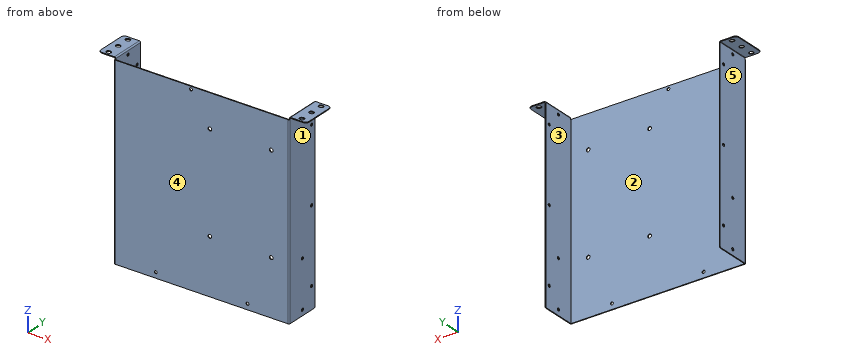
```python
from build123d import *

# Parameters (mm, degrees)
SKETCH1_W                    = 214
SKETCH1_H                    = 230.5
BASE_FLANGE1_DEPTH           = 1
EDGE_FLANGE3_STRIP_W         = 5
EDGE_FLANGE3_STRIP_H         = 1
EDGE_FLANGE3_STRIP_CUT_DEPTH = 230.5
EDGE_FLANGE3_DEPTH           = 230.5
EDGE_FLANGE4_STRIP_W         = 5
EDGE_FLANGE4_STRIP_H         = 1
EDGE_FLANGE4_STRIP_CUT_DEPTH = 230.5
EDGE_FLANGE4_DEPTH           = 230.5
EDGE_FLANGE5_STRIP_W         = 5
EDGE_FLANGE5_STRIP_H         = 1
EDGE_FLANGE5_STRIP_CUT_DEPTH = 41.5
EDGE_FLANGE5_DEPTH           = 41.5
EDGE_FLANGE6_STRIP_W         = 5
EDGE_FLANGE6_STRIP_H         = 1
EDGE_FLANGE6_STRIP_CUT_DEPTH = 41.5
EDGE_FLANGE6_DEPTH           = 41.5
FILLET1_R                    = 4
CUT_EXTRUDE1_REACH           = 178.807
SKETCH24_W                   = 214
SKETCH24_H                   = 2.5
SKETCH26_R                   = 2.5
CUT_EXTRUDE2_DEPTH           = 10
SKETCH27_R                   = 1.75
CUT_EXTRUDE3_DEPTH           = 265.201745831
SKETCH28_R                   = 2.25
CUT_EXTRUDE4_DEPTH           = 177.806568034
SKETCH29_R                   = 1.75
CUT_EXTRUDE5_DEPTH           = 177.566028726
SKETCH30_R                   = 1.75
CUT_EXTRUDE6_DEPTH           = 265.201745831
SKETCH31_R                   = 1.75
CUT_EXTRUDE7_DEPTH           = 265.201745831
CHAMFER1_SIZE                = 1
CUT_EXTRUDE8_DEPTH           = 266.637440885
SKETCH33_R                   = 1.75
CUT_EXTRUDE9_DEPTH           = 177.806568034
SKETCH34_R                   = 1.75
CUT_EXTRUDE10_DEPTH          = 265.201745831


# Sheet-metal steps are written as plain solids
with BuildPart() as part:
    # Sketch1 → Base-Flange1 (new body)
    with BuildSketch(Plane(origin=(0, 0, 0), x_dir=(1, 0, 0), z_dir=(0, 1, 0))):
        Rectangle(SKETCH1_W, SKETCH1_H)
    extrude(amount=-BASE_FLANGE1_DEPTH)

    # Edge-Flange3 strip (across the edge) → Edge-Flange3 strip cut (cut)
    with BuildSketch(Plane(origin=(-107, 0, -115.25), x_dir=(1, 0, 0), z_dir=(0, 0, 1))):
        with Locations((-1, -0.5)):
            Rectangle(EDGE_FLANGE3_STRIP_W, EDGE_FLANGE3_STRIP_H)
    extrude(amount=EDGE_FLANGE3_STRIP_CUT_DEPTH, mode=Mode.SUBTRACT)

    # Edge-Flange3 section (across the edge) → Edge-Flange3 (add)
    with BuildSketch(Plane(origin=(-107, 0, -115.25), x_dir=(1, 0, 0), z_dir=(0, 0, 1))):
        with BuildLine():
            Line((0, 0.5), (0, 42))
            Line((0, 42), (1, 42))
            Line((1, 42), (1, 0.5))
            ThreePointArc((1, 0.5), (1.146446609, 0.146446609), (1.5, 0))
            Line((1.5, 0), (1.5, -1))
            ThreePointArc((1.5, -1), (0.439339828, -0.560660172), (0, 0.5))
        make_face()
    extrude(amount=EDGE_FLANGE3_DEPTH)

    # Edge-Flange4 strip (across the edge) → Edge-Flange4 strip cut (cut)
    with BuildSketch(Plane(origin=(107, 0, 115.25), x_dir=(-1, 0, 0), z_dir=(0, 0, -1))):
        with Locations((-1, -0.5)):
            Rectangle(EDGE_FLANGE4_STRIP_W, EDGE_FLANGE4_STRIP_H)
    extrude(amount=EDGE_FLANGE4_STRIP_CUT_DEPTH, mode=Mode.SUBTRACT)

    # Edge-Flange4 section (across the edge) → Edge-Flange4 (add)
    with BuildSketch(Plane(origin=(107, 0, 115.25), x_dir=(-1, 0, 0), z_dir=(0, 0, -1))):
        with BuildLine():
            Line((0, 0.5), (0, 42))
            Line((0, 42), (1, 42))
            Line((1, 42), (1, 0.5))
            ThreePointArc((1, 0.5), (1.146446609, 0.146446609), (1.5, 0))
            Line((1.5, 0), (1.5, -1))
            ThreePointArc((1.5, -1), (0.439339828, -0.560660172), (0, 0.5))
        make_face()
    extrude(amount=EDGE_FLANGE4_DEPTH)

    # Edge-Flange5 strip (across the edge) → Edge-Flange5 strip cut (cut)
    with BuildSketch(Plane(origin=(107, 42, 115.25), x_dir=(0, 0, -1), z_dir=(0, -1, 0))):
        with Locations((-1, -0.5)):
            Rectangle(EDGE_FLANGE5_STRIP_W, EDGE_FLANGE5_STRIP_H)
    extrude(amount=EDGE_FLANGE5_STRIP_CUT_DEPTH, mode=Mode.SUBTRACT)

    # Edge-Flange5 section (across the edge) → Edge-Flange5 (add)
    with BuildSketch(Plane(origin=(107, 42, 115.25), x_dir=(0, 0, -1), z_dir=(0, -1, 0))):
        with BuildLine():
            Line((0, 0.5), (0, 20))
            Line((0, 20), (1, 20))
            Line((1, 20), (1, 0.5))
            ThreePointArc((1, 0.5), (1.146446609, 0.146446609), (1.5, 0))
            Line((1.5, 0), (1.5, -1))
            ThreePointArc((1.5, -1), (0.439339828, -0.560660172), (0, 0.5))
        make_face()
    extrude(amount=EDGE_FLANGE5_DEPTH)

    # Edge-Flange6 strip (across the edge) → Edge-Flange6 strip cut (cut)
    with BuildSketch(Plane(origin=(-107, 0.5, 115.25), x_dir=(0, 0, -1), z_dir=(0, 1, 0))):
        with Locations((-1, -0.5)):
            Rectangle(EDGE_FLANGE6_STRIP_W, EDGE_FLANGE6_STRIP_H)
    extrude(amount=EDGE_FLANGE6_STRIP_CUT_DEPTH, mode=Mode.SUBTRACT)

    # Edge-Flange6 section (across the edge) → Edge-Flange6 (add)
    with BuildSketch(Plane(origin=(-107, 0.5, 115.25), x_dir=(0, 0, -1), z_dir=(0, 1, 0))):
        with BuildLine():
            Line((0, 0.5), (0, 20))
            Line((0, 20), (1, 20))
            Line((1, 20), (1, 0.5))
            ThreePointArc((1, 0.5), (1.146446609, 0.146446609), (1.5, 0))
            Line((1.5, 0), (1.5, -1))
            ThreePointArc((1.5, -1), (0.439339828, -0.560660172), (0, 0.5))
        make_face()
    extrude(amount=EDGE_FLANGE6_DEPTH)

    # Fillet1
    fillet1_edges = [part.edges().sort_by_distance(p)[0] for p in [
        (127, 42, 114.75),
        (127, 0.5, 114.75),
        (-127, 0.5, 114.75),
        (-127, 42, 114.75),
    ]]
    fillet(fillet1_edges, radius=FILLET1_R)

    # Cut-Extrude1: up to this face of the body (flat: up to its plane)
    cut_extrude1_end = Plane(part.part.faces().sort_by_distance((114.980552593, 0.5, 114.747536063))[0])
    # Sketch24 → Cut-Extrude1 (cut, up to the picked face)
    with BuildSketch(Plane.XZ.offset(1), mode=Mode.PRIVATE) as cut_extrude1_sk1:
        with Locations((0, 114)):
            Rectangle(SKETCH24_W, SKETCH24_H)
    cut_extrude1_tool1 = split(extrude(cut_extrude1_sk1.sketch, amount=-CUT_EXTRUDE1_REACH, mode=Mode.PRIVATE), bisect_by=cut_extrude1_end, keep=Keep.BOTH, mode=Mode.PRIVATE)
    add(cut_extrude1_tool1.solids().sort_by(Axis((0, -1, 114), (0, 1, 0)))[0], mode=Mode.SUBTRACT)

    # Sketch26 → Cut-Extrude2 (cut)
    with BuildSketch(Plane.XY.offset(115.25)):
        with Locations((-118, 37)):
            Circle(SKETCH26_R)
        with Locations((-118, 5.24)):
            Circle(SKETCH26_R)
        with Locations((-118, 21.12)):
            Circle(SKETCH26_R)
        with Locations(Location((118, 5.24, 0), (0, 0, 180))):
            Circle(SKETCH26_R)
        with Locations(Location((118, 21.12, 0), (0, 0, 180))):
            Circle(SKETCH26_R)
        with Locations(Location((118, 37, 0), (0, 0, 180))):
            Circle(SKETCH26_R)
    extrude(amount=-CUT_EXTRUDE2_DEPTH, mode=Mode.SUBTRACT)

    # Sketch27 → Cut-Extrude3 (cut, through all)
    with BuildSketch(Plane(origin=(107, 0, 0), x_dir=(0, 0, -1), z_dir=(1, 0, 0))):
        with Locations(Location((-91.5, 36.25, 0), (0, 0, 90))):
            Circle(SKETCH27_R)
        with Locations(Location((-1.5, 36.25, 0), (0, 0, 90))):
            Circle(SKETCH27_R)
        with Locations(Location((88.5, 36.25, 0), (0, 0, 90))):
            Circle(SKETCH27_R)
    extrude(amount=-CUT_EXTRUDE3_DEPTH, mode=Mode.SUBTRACT)

    # Sketch28 → Cut-Extrude4 (cut, through all)
    with BuildSketch(Plane.XZ.offset(1)):
        with Locations(Location((10, 72.25, 0), (0, 0, 270))):
            Circle(SKETCH28_R)
        with Locations(Location((85, 72.25, 0), (0, 0, 270))):
            Circle(SKETCH28_R)
        with Locations(Location((10, -47.75, 0), (0, 0, 270))):
            Circle(SKETCH28_R)
        with Locations(Location((85, -47.75, 0), (0, 0, 270))):
            Circle(SKETCH28_R)
    extrude(amount=-CUT_EXTRUDE4_DEPTH, mode=Mode.SUBTRACT)

    # Sketch29 → Cut-Extrude5 (cut, through all)
    with BuildSketch(Plane(origin=(0, 0, 0), x_dir=(1, 0, 0), z_dir=(0, 1, 0))):
        with Locations(Location((56, 108.45, 0), (0, 0, 270))):
            Circle(SKETCH29_R)
        with Locations(Location((-56, 108.45, 0), (0, 0, 270))):
            Circle(SKETCH29_R)
    extrude(amount=-CUT_EXTRUDE5_DEPTH, mode=Mode.SUBTRACT)

    # Sketch30 → Cut-Extrude6 (cut, through all)
    with BuildSketch(Plane.ZY.offset(107)):
        with Locations(Location((-51.1, 21, 0), (0, 0, 270))):
            Circle(SKETCH30_R)
    extrude(amount=-CUT_EXTRUDE6_DEPTH, mode=Mode.SUBTRACT)

    # Sketch31 → Cut-Extrude7 (cut, through all)
    with BuildSketch(Plane.ZY.offset(107)):
        with Locations(Location((-108.45, 21, 0), (0, 0, 270))):
            Circle(SKETCH31_R)
    extrude(amount=-CUT_EXTRUDE7_DEPTH, mode=Mode.SUBTRACT)

    # Chamfer1
    chamfer1_edges = [part.edges().sort_by_distance(p)[0] for p in [
        (-106.5, 42, -115.25),
        (106.5, 42, -115.25),
    ]]
    chamfer(chamfer1_edges, length=CHAMFER1_SIZE)

    # Sketch32 → Cut-Extrude8 (cut, through all)
    with BuildSketch(Plane(origin=(0, 0, 114.25), x_dir=(-1, 0, 0), z_dir=(0, 0, -1))):
        with BuildLine():
            Line((117.5, 39.5), (118.5, 39.5))
            ThreePointArc((118.5, 39.5), (121, 37), (118.5, 34.5))
            Line((118.5, 34.5), (117.5, 34.5))
            ThreePointArc((117.5, 34.5), (115, 37), (117.5, 39.5))
        make_face()
        with BuildLine():
            Line((117.5, 23.62), (118.5, 23.62))
            ThreePointArc((118.5, 23.62), (121, 21.12), (118.5, 18.62))
            Line((118.5, 18.62), (117.5, 18.62))
            ThreePointArc((117.5, 18.62), (115, 21.12), (117.5, 23.62))
        make_face()
        with BuildLine():
            Line((117.5, 7.74), (118.5, 7.74))
            ThreePointArc((118.5, 7.74), (121, 5.24), (118.5, 2.74))
            Line((118.5, 2.74), (117.5, 2.74))
            ThreePointArc((117.5, 2.74), (115, 5.24), (117.5, 7.74))
        make_face()
    cut_extrude8 = extrude(amount=-CUT_EXTRUDE8_DEPTH, mode=Mode.SUBTRACT)

    # Mirror1: Cut-Extrude8 across plane
    add(cut_extrude8.mirror(Plane(origin=(0, 0, 0), x_dir=(0, 0, 1), z_dir=(1, 0, 0))), mode=Mode.SUBTRACT)

    # Sketch33 → Cut-Extrude9 (cut, through all)
    with BuildSketch(Plane.XZ.offset(1)):
        with Locations(Location((-13, 109.25, 0), (0, 0, 270))):
            Circle(SKETCH33_R)
    extrude(amount=-CUT_EXTRUDE9_DEPTH, mode=Mode.SUBTRACT)

    # Sketch34 → Cut-Extrude10 (cut, through all)
    with BuildSketch(Plane.ZY.offset(107)):
        with Locations(Location((109.25, 21, 0), (0, 0, 270))):
            Circle(SKETCH34_R)
    extrude(amount=-CUT_EXTRUDE10_DEPTH, mode=Mode.SUBTRACT)


solid = part.part
```
Geometry: final body of the model. Coordinates: model frame, mm. Face numbers are marked on the shaded views. A direction names the side the tool comes from. Round coordinates to 2 decimals unless told otherwise and drop trailing zeros. Loops run counter-clockwise (first coordinate to the right, second up) from the corner with the lowest first, then second, coordinate; pieces in that order, holes last. Notation, with made-up numbers: (-32.75, -20.5) -> (-11.75, -20.5) arc R28 ccw to (-11.75, -2.5) -> close; hole circle Ø6 at (89, -5.75). An arc over 180 degrees is marked (long way). Use one line per item in the form item = value. Start each with the question number.
1) Line query: L1, parallel to X at y = 26, z = 84.5; L2, parallel to Z at x = 106.6, y = 36.25; L3, parallel to Y at x = -98.5, z = -77.5. Output: solid intervals per line, ascending.
2) First-contact query: P1, Ø4, axis at y = 21.5, z = 32.5, coming from the +X side; P2, Ø6, axis at x = 10, z = 72.25, coming from the +Y side; P3, Ø5.5, axis at y = 21, z = -51.1, coming from the -X side. Flat tips, straight axial feed; report the tip coordinate or a pass-through.
3) Section C-C on x = 37. Output: boundary loops of the cut face in (y, z), then the cut area to 3 significant figures.
4) Access query for the marked faces 1 and 2. Directions: +Z, -Z, +X, -X, +Y, -Y. A direction counts if a zero-diameter tool reaches every point of the face in a straight line with its end or side. Return the directions, or none.
5) Section A-A on y = 29. Output: boundary loops of the cut face in (x, z), then the cut area to 3 significant figures.
6) Draft query along X for the marked faces 3, 4 and 5. Return one class per face: released by +X, released by -X, zero draft, split by the parting line, or undercut.
7) Section B-B on z = 37. Output: boundary loops of the cut face in (x, y), then the cut area to 3 significant figures.
Response:
q1.L1 = -107 to -106, 106 to 107
q1.L2 = -115.25 to -90.25, -86.75 to -0.25, 3.25 to 89.75, 93.25 to 114.95
q1.L3 = -1 to 0
q2.P1 = 107
q2.P2 = 0
q2.P3 = -107
q3.outline = (-1, -115.25) -> (0, -115.25) -> (0, 112.75) -> (-1, 112.75) -> close
q3.area = 228 mm^2
q4.face_1 = -Z, +X, +Y, -Y
q4.face_2 = +Z, -Z, +Y
q5.outline = (-127, 114.25) -> (-107.5, 114.25) arc R0.5 cw to (-107, 113.75) -> (-107, -115.25) -> (-106, -115.25) -> (-106, 113.75) arc R1.5 ccw to (-107.5, 115.25) -> (-127, 115.25) -> close; (106, -115.25) -> (107, -115.25) -> (107, 113.75) arc R0.5 cw to (107.5, 114.25) -> (127, 114.25) -> (127, 115.25) -> (107.5, 115.25) arc R1.5 ccw to (106, 113.75) -> close
q5.area = 500 mm^2
q6.face_3 = undercut
q6.face_4 = zero draft
q6.face_5 = released by -X
q7.outline = (-107, 0.5) arc R1.5 ccw to (-105.5, -1) -> (105.5, -1) arc R1.5 ccw to (107, 0.5) -> (107, 42) -> (106, 42) -> (106, 0.5) arc R0.5 cw to (105.5, 0) -> (-105.5, 0) arc R0.5 cw to (-106, 0.5) -> (-106, 42) -> (-107, 42) -> close
q7.area = 297 mm^2
